Design review of the part shown in the three views and the two pictorial views. Dimensions are in mm from the part's minimum x, y and z. A direction names the side the tool comes from. Coordinates: 2 decimals unless noted, no trailing zeros. Loops run counter-clockwise (first coordinate to the right, second up) from the corner with the lowest first, then second, coordinate; pieces in that order, holes last. Notation, with made-up numbers: (71, -28.75) -> (100, -28.75) arc R25 ccw to (100, -3.75) -> close; hole circle Ø10 at (45.5, -10.5). An arc over 180 degrees is marked (long way). One line per item, written item: value.
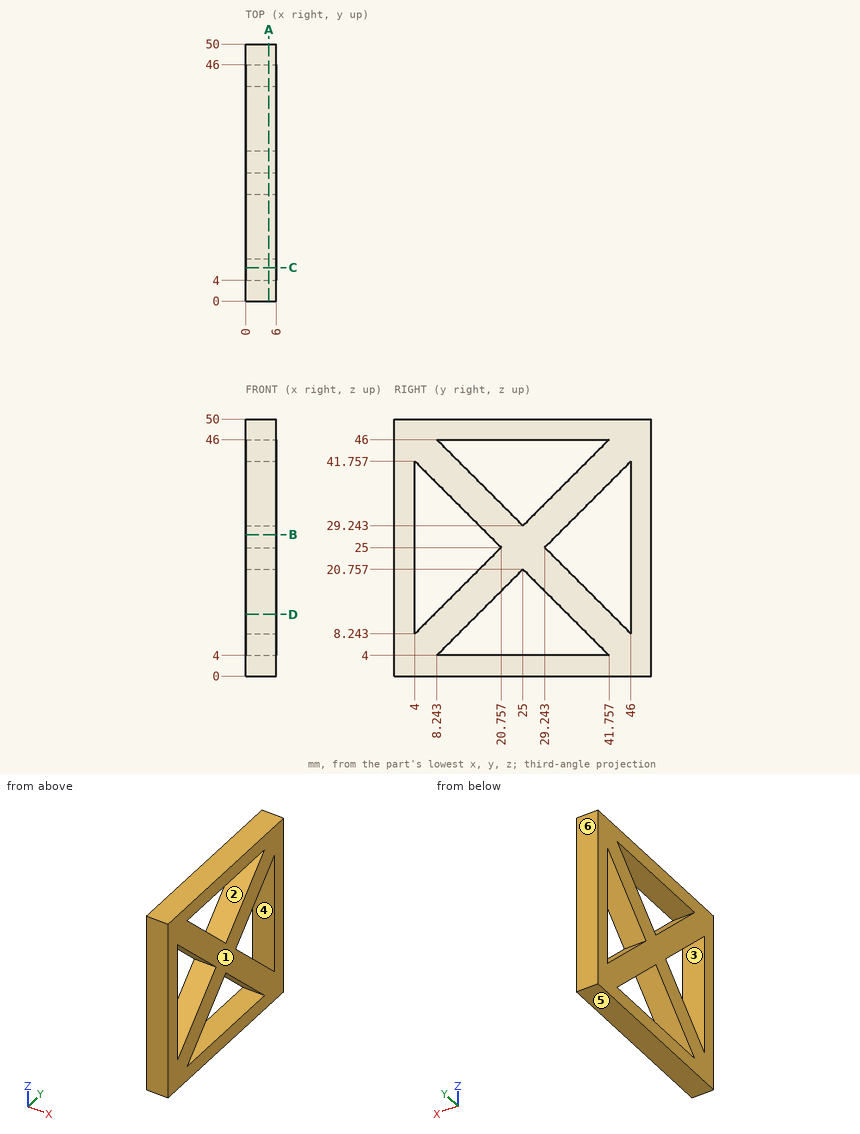
1. To check wall thickness, follow probe 1 along Z at (x, y) = (2.5, 35); probe 2 along Y at (x, z) = (3.15, 39.5); probe 3 along Y at (x, z) = (4.2, 24.5). State the ranges of each line that lie inside material, in increasing order. Write a range as from..to.
Return value:
probe 1: z = 0..4, 10.76..19.24, 30.76..39.24, 46..50
probe 2: y = 0..4, 6.26..14.74, 35.26..43.74, 46..50
probe 3: y = 0..4, 20.26..29.74, 46..50
2. The part is to be moulded in two halves that separate along Z. For the marked faces 3, 4, 5 and 6, say which applies: pulls with the +Z half, pulls with the -Z half, needs draft (parallel to the pull), parting line crosses it, or undercut.
Return value:
face 3: undercut
face 4: undercut
face 5: pulls with the -Z half
face 6: needs draft
3. Take a section at B-B, the plane z = 27.5. Give the boundary of the cut face in (x, y).
Return value:
outline: (0, 0) -> (6, 0) -> (6, 4) -> (0, 4) -> close; (0, 18.26) -> (6, 18.26) -> (6, 31.74) -> (0, 31.74) -> close; (0, 46) -> (6, 46) -> (6, 50) -> (0, 50) -> close
4. Take a section at D-D, the plane z = 12. Give the boundary of the cut face in (x, y).
Return value:
outline: (0, 0) -> (6, 0) -> (6, 4) -> (0, 4) -> close; (0, 7.76) -> (6, 7.76) -> (6, 16.24) -> (0, 16.24) -> close; (0, 33.76) -> (6, 33.76) -> (6, 42.24) -> (0, 42.24) -> close; (0, 46) -> (6, 46) -> (6, 50) -> (0, 50) -> close
5. For the marked faces 1 and 2, list the 3-axis set-ups (+Z, -Z, +X, -X, +Y, -Y) from which the entire face can be reached by the end or side of a thin tool; tool diameter is ignored.
Return value:
face 1: +Z, -Z, +X, +Y, -Y
face 2: +X, -X
6. Take a section at C-C, the plane y = 6.5. Give the boundary of the cut face in (x, z).
Return value:
outline: (0, 0) -> (6, 0) -> (6, 10.74) -> (0, 10.74) -> close; (0, 39.26) -> (6, 39.26) -> (6, 50) -> (0, 50) -> close
7. Take a section at A-A, the plane x = 4.55. Give the boundary of the cut face in (y, z), and give its area (3 significant figures).
Return value:
outline: (0, 0) -> (50, 0) -> (50, 50) -> (0, 50) -> close; hole (4, 8.24) -> (20.76, 25) -> (4, 41.76) -> close; hole (8.24, 4) -> (41.76, 4) -> (25, 20.76) -> close; hole (8.24, 46) -> (25, 29.24) -> (41.76, 46) -> close; hole (29.24, 25) -> (46, 8.24) -> (46, 41.76) -> close
area: 1,380 mm2
